Autodesk Inventor part; units mm, degrees
ref_plane "YZ Plane" through (0, 0, 0) normal (1, 0, 0) x (0, 1, 0)
ref_plane "XZ Plane" through (0, 0, 0) normal (0, 1, 0) x (-1, 0, 0)
ref_plane "XY Plane" through (0, 0, 0) normal (0, 0, 1) x (1, 0, 0)
sketch "Эскиз1" plane through (0, 0, 0) normal (0, 1, 0) x (-1, 0, 0)
  arc A0 (8.8038, -3) -> (8.8038, 3) centre (14, 0) ccw
  line L0 (30.0057, 0) -> (28.0258, 0)
  circle A1 centre (14, 0) radius 1.9
  arc A2 (-8.8038, 3) -> (-8.8038, -3) centre (-14, 0) ccw
  line L1 (-8.8038, -3) -> (8.8038, -3)
  line L2 (-8.8038, 3) -> (8.8038, 3)
  circle A3 centre (-14, 0) radius 1.9
  line L3 (32.9518, 0) -> (37.6343, 0) construction
  line L4 (14.11, -3) -> (14.11, 3)
  line L5 (0, -3) -> (0, 3)
  point P0 (0, 0)
  point P1 (25.2378, -3)
  point P2 (25.2378, 3)
  point P3 (0, 0)
  dimension "d2" = 6
  dimension "d3" = 14
  dimension "d4" = 3.8
  dimension "d9" = 6
extrude "Выдавливание1" add sketch "Эскиз1" along normal mid plane 3
fillet "Сопряжение1" radius 10 4 edges at (-8.8038, 0, 3) (-8.8038, 0, -3) (8.8038, 0, -3) (8.8038, 0, 3)
properties part number "Рычаг"
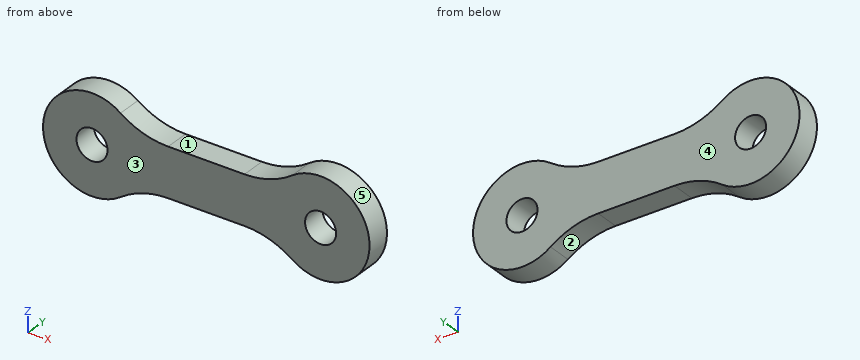
Geometry check sheet. Reference: the model listing, model coordinates, mm. Face numbers are marked on the shaded views. A direction names the side the tool comes from. Give positions to 0.01 mm unless a question says otherwise; leave off trailing zeros. Order: outer loops, then holes, each group sorted by start corner. A loop starts at its lowest first (then second) coordinate and runs counter-clockwise, first axis right, second up.
1. Release check for a two-part mould opening along X. For the marked faces 4 and 5 record: pulls with the +X half, pulls with the -X half, needs draft (parallel to the pull), parting line crosses it, or undercut.
2. Thickness scan on L1, parallel to Z at x = -14, y = 0.6; L2, parallel to X at y = 1.2, z = -1.5; L3, parallel to X at y = 0.45, z = 0.75. Record the ranges inside material, lowest first.
3. Gauge pin test, flat ends, axial feed: pin 1 Ø1 at (x, y) = (-0.5, 1) entering from -Z; pin 2 Ø1 at (y, z) = (1, -1) entering from -X; pin 3 Ø0.9 at (x, y) = (-1, 0.5) entering from +Z. Record the tip position at first contact, or that the pin passes through.
4. Section check B-B, the plane x = 14. Enter the section's corners in (y, z).
5. Access from +Z, -Z, +X, -X, +Y, -Y to the whole of each face (thin tool, end or side, straight path). Record for the marked faces 1, 2 and 3.
6. Section check C-C, the plane y = -0.95. Enter the section's corners in (x, z), and give its area (3 significant figures).
7. Section check D-D, the plane z = 3.5. Enter the section's corners in (x, y).
8. Section check A-A, the plane z = 0. Enter the section's corners in (x, y).
Values follow:
1. face 4: needs draft
1. face 5: undercut
2. L1: z = -6 to -1.9, 1.9 to 6
2. L2: x = -19.81 to -15.17, -12.83 to 12.83, 15.17 to 19.81
2. L3: x = -19.95 to -15.75, -12.25 to 12.25, 15.75 to 19.95
3. pin 1: stops at z = -3
3. pin 2: stops at x = -19.98
3. pin 3: stops at z = 3
4. outline: (-1.5, -6) - (1.5, -6) - (1.5, -1.9) - (-1.5, -1.9) - close; (-1.5, 1.9) - (1.5, 1.9) - (1.5, 6) - (-1.5, 6) - close
5. face 1: +Z, +Y, -Y
5. face 2: -Z, +Y, -Y
5. face 3: +Z, -Z, +X, -X, -Y
6. outline: (-10.5, -4.88) arc R10 cw to (-4.67, -3) - (4.67, -3) arc R10 cw to (10.5, -4.88) arc R6 ccw (long way) to (10.5, 4.88) arc R10 cw to (4.67, 3) - (-4.67, 3) arc R10 cw to (-10.5, 4.88) arc R6 ccw (long way) to start; hole circle Ø3.8 at (-14, 0); hole circle Ø3.8 at (14, 0)
6. area: 309 mm2
7. outline: (-18.87, -1.5) - (-7.8, -1.5) - (-7.8, 1.5) - (-18.87, 1.5) - close; (7.8, -1.5) - (18.87, -1.5) - (18.87, 1.5) - (7.8, 1.5) - close
8. outline: (-20, -1.5) - (-15.9, -1.5) - (-15.9, 1.5) - (-20, 1.5) - close; (-12.1, -1.5) - (12.1, -1.5) - (12.1, 1.5) - (-12.1, 1.5) - close; (15.9, -1.5) - (20, -1.5) - (20, 1.5) - (15.9, 1.5) - close
